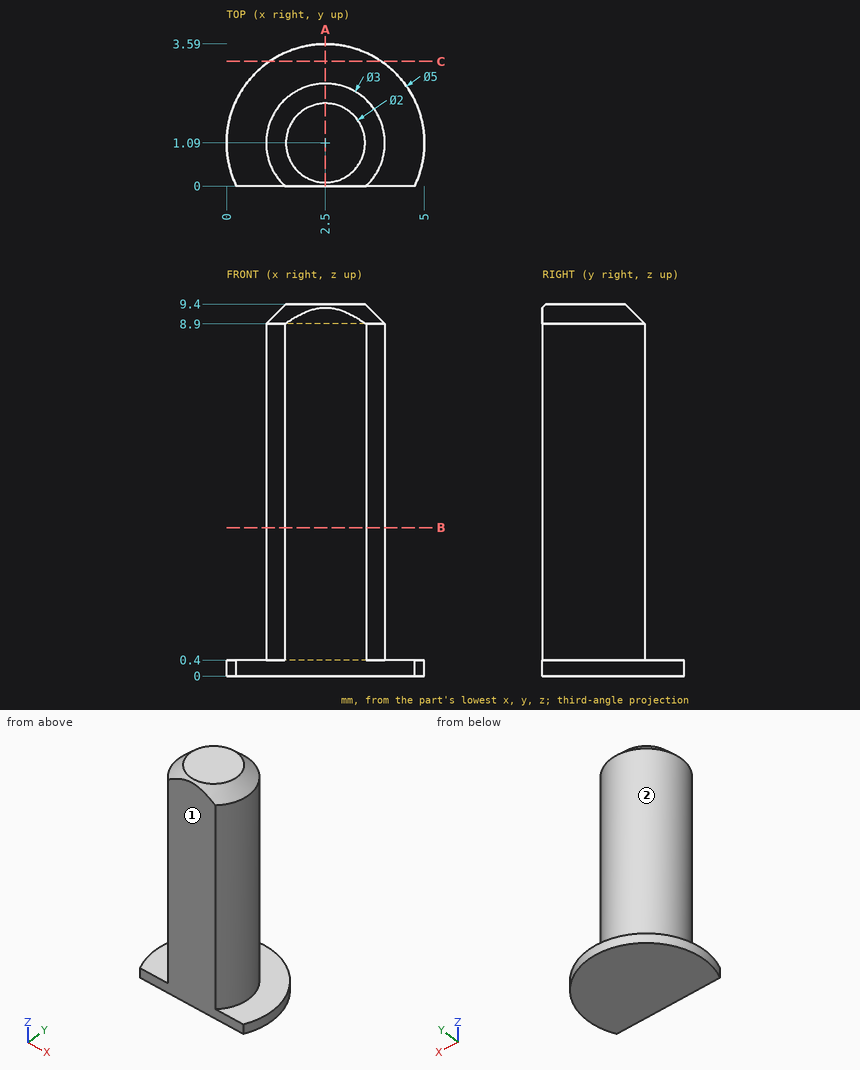
Print and shaded views of the part. All mm, measured from the part's lowest x, y and z. A direction names the side the tool comes from. Coordinates: 2 decimals unless noted, no trailing zeros. Loops run counter-clockwise (first coordinate to the right, second up) from the corner with the lowest first, then second, coordinate; pieces in that order, holes last. Notation, with made-up numbers: (13.5, -11) - (52.5, -11) arc R26 cw to (52.5, 14) - close; hole circle Ø1 at (-19, 80.5). An arc over 180 degrees is marked (long way). Use one line per item in the form item = value. Start each with the question number.
1) Tool access for the marked faces 1 and 2: list every direction of +Z, -Z, +X, -X, +Y, -Y with a clear straight run to the whole face (end or side of a thin tool).
2) Band-saw the part on B-B (z = 3.75). Give the cut face in (x, y).
3) Band-saw the part on C-C (y = 3.15). Give the cut face in (x, z).
4) Flat gauge pins, fed straight in: pin 1 (2 mm diameter, centred on x = 4, z = 4.5, fed in from +Y); pin 2 (1 mm diameter, centred on x = 3, z = 5, fed in from +Y); pin 3 (2 mm diameter, centred on y = 3, z = 4.5, fed in from +X). Where does each tip first touch, or does it go through?
5) Drill centre lines: L1, parallel to Z at x = 3.6, y = 2.55; L2, parallel to X at y = 1.15, z = 4; L3, parallel to Y at x = 3.4, z = 4.5. Where is each one in solid material? Low to high. Write a range as from..to.
6) Band-saw the part on A-A (x = 2.5). Give the cut face in (y, z).
Check values:
q1.face_1 = +Z, -Z, +X, -X, -Y
q1.face_2 = +Z
q2.outline = (1.47, 0) - (3.53, 0) arc R1.5 ccw (long way) to start
q3.outline = (1.08, 0) - (3.92, 0) - (3.92, 0.4) - (1.08, 0.4) - close
q4.pin_1 = 2.5
q4.pin_2 = 2.59
q4.pin_3 = 3.69
q5.L1 = 0..0.4
q5.L2 = 1..4
q5.L3 = 0..2.29
q6.outline = (0, 0) - (3.59, 0) - (3.59, 0.4) - (2.59, 0.4) - (2.59, 8.9) - (2.09, 9.4) - (0.09, 9.4) - (0, 9.31) - close
